from build123d import *

# Parameters (mm, degrees)
F0_W     = 58.42
F0_H     = 124.46
F1_DEPTH = 25.4
F2_W     = 49.598961
F2_H     = 51.409137
F2_H_2   = 43.945098
F2_H_3   = 11.481412
F3_DEPTH = 20.32
F4_R     = 5.08
F5_W     = 18.630186
F5_H     = 46.435684
F6_DEPTH = 12.7
F7_R     = 8.89


with BuildPart() as f1:
    # F0 (on Top) → F1 (new body)
    with BuildSketch(Plane.XY):
        with Locations((-18.543279, 2.624761)):
            Rectangle(F0_W, F0_H)
    extrude(amount=F1_DEPTH)

    # F2 (on face) → F3 (cut)
    with BuildSketch(Plane.XY.offset(25.4)):
        with Locations((-19.09741, 33.035801)):
            Rectangle(F2_W, F2_H)
        with Locations((-19.09741, -19.347788)):
            Rectangle(F2_W, F2_H_2)
        with Locations((-19.09741, -49.922362)):
            Rectangle(F2_W, F2_H_3)
    extrude(amount=-F3_DEPTH, mode=Mode.SUBTRACT)

    # F4
    f4_edges = [f1.edges().sort_by_distance(p)[0] for p in [
        (5.70207, 58.74037, 15.24),
        (-43.896891, 58.74037, 15.24),
        (-43.896891, 7.331233, 15.24),
        (5.70207, 7.331233, 15.24),
        (-43.896891, 2.624761, 15.24),
        (5.70207, 2.624761, 15.24),
        (5.70207, -41.320337, 15.24),
        (-43.896891, -41.320337, 15.24),
        (5.70207, -44.181656, 15.24),
        (5.70207, -55.663068, 15.24),
        (-43.896891, -44.181656, 15.24),
        (-43.896891, -55.663068, 15.24),
    ]]
    fillet(f4_edges, radius=F4_R)

    # F5 (on face) → F6 (cut)
    with BuildSketch(Plane.XY.offset(25.4)):
        with Locations((-19.545062, -9.993736)):
            Rectangle(F5_W, F5_H)
    extrude(amount=-F6_DEPTH, mode=Mode.SUBTRACT)

    # F7
    f7_edges = [f1.edges().sort_by_distance(p)[0] for p in [
        (-10.229969, 4.977997, 12.7),
        (-28.860155, 4.977997, 12.7),
    ]]
    fillet(f7_edges, radius=F7_R)


solid = f1.part
The listing builds one solid part. Answer for the finished solid, in the listing's coordinates (mm). A direction names the side the tool comes from. Give positions to 0.01 mm unless a question says otherwise; leave off trailing zeros. Write each loop counter-clockwise with the first axis right and the second up, starting at its lowest first coordinate (ties: lowest second). Pieces come first, ordered by that corner, then holes. Notation, with made-up numbers: (31.25, -18) - (49.25, -18) arc R21 cw to (49.25, 6) - close; hole circle Ø1 at (-23.75, -35.5). An arc over 180 degrees is marked (long way). Use a Markdown table: item, result.
1. Section C-C on x = -37.5 is taken. Write down the section's boundary in (y, z).
Values follow:
| item | result |
|---|---|
| outline | (-59.61, 0) - (64.85, 0) - (64.85, 25.4) - (58.74, 25.4) - (58.74, 5.08) - (7.33, 5.08) - (7.33, 25.4) - (2.62, 25.4) - (2.62, 5.08) - (-41.32, 5.08) - (-41.32, 25.4) - (-44.18, 25.4) - (-44.18, 5.08) - (-55.66, 5.08) - (-55.66, 25.4) - (-59.61, 25.4) - close |
2. Section D-D on z = 19.75 is taken. Count the separate pieces of the cut face and the enclosed holes in it, plus the area to 3 significant figures.
Values follow:
| item | result |
|---|---|
| separate pieces | 1 |
| enclosed holes | 2 |
| area | 1,950 mm² |
3. For a pull along X with two mould halves and no side action, classify faces 3 (the flat face through (-47.753, 2, 13)), 4 (the cylindrical face through (4.25, 1.1, 15.1)), 5 (the flat face through (-19, 64.855, 13)), 6 (the flat face through (-43.897, 33, 15)) as released by +X, released by -X, zero draft, split by the parting line, or undercut.
Values follow:
| item | result |
|---|---|
| face 3 | released by -X |
| face 4 | undercut |
| face 5 | zero draft |
| face 6 | undercut |
4. Section B-B on y = -13 is taken. Write down the section's boundary in (x, z), plus the area to 3 significant figures.
Values follow:
| item | result |
|---|---|
| outline | (-47.75, 0) - (10.67, 0) - (10.67, 25.4) - (5.7, 25.4) - (5.7, 5.08) - (-43.9, 5.08) - (-43.9, 25.4) - (-47.75, 25.4) - close |
| area | 476 mm² |
5. Find the intervals of material crossed by probe 1 along Y at (x, z) = (-18, 14); probe 2 along Y at (x, z) = (-31.5, 12.25); probe 3 along X at (y, z) = (-32, 9), in increasing order. Write a range as from..to.
Values follow:
| item | result |
|---|---|
| probe 1 | y = -59.61..-55.66, -44.18..-41.32, 58.74..64.85 |
| probe 2 | y = -59.61..-55.66, -44.18..-41.32, 2.62..7.33, 58.74..64.85 |
| probe 3 | x = -47.75..-43.9, 5.7..10.67 |
6. Each of these flat-tipped pins is pushed along its axis until it touches: P1, Ø2, axis at x = -31.5, y = 44, coming from the +Z side; P2, Ø0.9, axis at x = -19.5, y = 5.5, coming from the +Z side. Where does it stop, or does it pass through?
Values follow:
| item | result |
|---|---|
| P1 | stops at z = 5.08 |
| P2 | stops at z = 12.7 |
7. Section A-A on z = 9.75 is taken. Write down the section's boundary in (x, y).
Values follow:
| item | result |
|---|---|
| outline | (-47.75, -59.61) - (10.67, -59.61) - (10.67, 64.85) - (-47.75, 64.85) - close; hole (-43.9, -50.58) arc R5.08 ccw to (-38.82, -55.66) - (0.62, -55.66) arc R5.08 ccw to (5.7, -50.58) - (5.7, -49.26) arc R5.08 ccw to (0.62, -44.18) - (-38.82, -44.18) arc R5.08 ccw to (-43.9, -49.26) - close; hole (-43.9, -36.24) arc R5.08 ccw to (-38.82, -41.32) - (0.62, -41.32) arc R5.08 ccw to (5.7, -36.24) - (5.7, -2.46) arc R5.08 ccw to (0.62, 2.62) - (-38.82, 2.62) arc R5.08 ccw to (-43.9, -2.46) - close; hole (-43.9, 12.41) arc R5.08 ccw to (-38.82, 7.33) - (0.62, 7.33) arc R5.08 ccw to (5.7, 12.41) - (5.7, 53.66) arc R5.08 ccw to (0.62, 58.74) - (-38.82, 58.74) arc R5.08 ccw to (-43.9, 53.66) - close |
8. A tool of negligible diameter and unlimited length cuts with its end or side. For faces 1 (the flat face through (-10, 3, 25.4)), 2 (the cylindrical face through (4.253, -45.709, 15.098)), from which of +Z, -Z, +X, -X, +Y, -Y can it reach the whole face along a straight path? Write none if from no direction.
Values follow:
| item | result |
|---|---|
| face 1 | +Z, +X, -X, +Y, -Y |
| face 2 | +Z |
